Check sheet for the modelled part. Datum: model origin and axes. Units: mm. Face numbers are marked on the shaded views. Round coordinates to 2 decimals unless told otherwise and drop trailing zeros. Order: outer loops, then holes, each group sorted by start corner. A loop starts at its lowest first (then second) coordinate and runs counter-clockwise, first axis right, second up.
```python
from build123d import *

# Parameters (mm, degrees)
BASENUT_START = -3.1
BASENUTSKE_R  = 1
BASENUT_DEPTH = 3.1


# Read off the part's stored shape, not the designer's step: ThreadSchematic
with BuildPart() as part:
    # BaseNutSke → BaseNut (new body)
    with BuildSketch(Plane.XY.offset(BASENUT_START)):
        Polygon((2.75, 1.58771324), (2.75, -1.58771324), (0, -3.175426481), (-2.75, -1.58771324), (-2.75, 1.58771324), (0, 3.175426481), align=None)
        Circle(BASENUTSKE_R, mode=Mode.SUBTRACT)
    extrude(amount=BASENUT_DEPTH)

    # Sketch5 (on Front Plane) → EndChamfer (revolve, cut)
    with BuildSketch(Plane.XY):
        Polygon((3.0746, 1.5), (2.689485854, 0.95), (3.1254, 0.95), (3.1254, 1.5), align=None)
    revolve(axis=Axis((3.1254, 0.95, 0), (-1, 0, 0)), mode=Mode.SUBTRACT)

    # Sketch3 → Double-Chamfer (revolve, cut)
    with BuildSketch(Plane(origin=(0, 0, 0), x_dir=(0, 0, -1), z_dir=(1, 0, 0)), mode=Mode.PRIVATE) as double_chamfer_sk:
        Polygon((3.1, 2.75), (2.854379907, 3.175426481), (2.854379907, 13.175426481), (13.1, 13.175426481), (13.1, 2.75), align=None)
        Polygon((0.95, 13.175426481), (-10, 13.175426481), (-10, 2.6125), (0, 2.6125), (0.95, 3.175426481), align=None)
    revolve(double_chamfer_sk.sketch.rotate(Axis((0, 0, 0), (0, 0, -1)), 300.000001719), axis=Axis((0, 0, 0), (0, 0, -1)), mode=Mode.SUBTRACT)

    # ThreadSchematic outline → ThreadSchematic (revolve, cut)
    with BuildSketch(Plane.XZ):
        Polygon((1, 0), (1, -0.350103769), (1.5, 0), align=None)
        Polygon((1.5, -3.0746), (1, -2.724496231), (1, -3.1), (1.5, -3.1), align=None)
    revolve(axis=Axis((0, 0, 0), (0, 0, 1)), mode=Mode.SUBTRACT)


solid = part.part
```
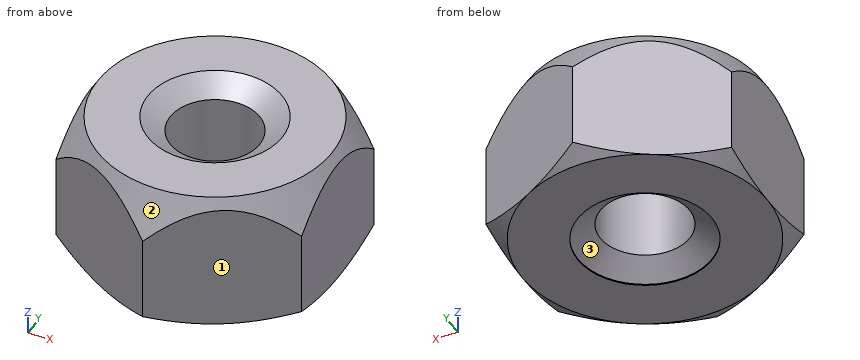
Item 1: Sectioned sample at A-A (z = -1.8). Record the cut outline in (x, y).
Answer:
outline: (-2.75, -1.59) - (0, -3.18) - (2.75, -1.59) - (2.75, 1.59) - (0, 3.18) - (-2.75, 1.59) - close; hole circle Ø2 at (0, 0)
Item 2: Go/stop test with a flat-tipped pin: P1, Ø2.5, axis at x = 0, y = 0, coming from the +Z side. Record where the tip stops, or that it passes through.
Answer:
P1: stops at z = -0.18
Item 3: Release check for a two-part mould opening along Y. For the marked faces 1, 2 and 3 record: released by +Y, released by -Y, zero draft, split by the parting line, or undercut.
Answer:
face 1: released by -Y
face 2: split by the parting line
face 3: undercut
Item 4: Scan lines: line 1 along Y through (x, z) = (0.75, -2.75); line 2 along Y through (x, z) = (0.85, -0.85); line 3 along Y through (x, z) = (-2.2, -2.3). Record each from-to range of solid material in increasing order.
Answer:
line 1: y = -2.74 to -0.72, 0.72 to 2.74
line 2: y = -2.68 to -0.53, 0.53 to 2.68
line 3: y = -1.91 to 1.91
